Verification items for the finished model (mm, model axes). A direction names the side the tool comes from. Give positions to 0.01 mm unless a question says otherwise; leave off trailing zeros. Order: outer loops, then holes, each group sorted by start corner. A loop starts at its lowest first (then second) coordinate and runs counter-clockwise, first axis right, second up. Notation, with made-up numbers: (89, 36.5) -> (107, 36.5) arc R22 ccw to (107, 43.5) -> close; hole circle Ø2 at (84, 49.5). An arc over 180 degrees is marked (long way). Return JSON: item names as keys, results as strings. Group by question number.
(1) Depth check by flat-ended pin: pin 1 Ø6 at (x, y) = (32, -4) entering from -Z; pin 2 Ø4 at (x, y) = (51, -23) entering from +Z; pin 3 Ø10 at (x, z) = (38.5, 26) entering from -Y; pin 4 Ø4 at (y, z) = (-9, 34) entering from -X. Enter the tip coordinate at first touch or a pass-through.
(2) Cross-section at C-C on y = -25. Enter the section's corners in (x, z), then the cut area to 3 significant figures.
(3) Tool access check on faces 1 (the face through (12, -17, 2.54)), 2 (the face through (58, 0, 49)). Record the directions out of +Z, -Z, +X, -X, +Y, -Y that give a thin tool (end or side, any length) a straight path to the whole face; none if there is none.
(4) Cross-section at B-B on z = 54. Enter the section's corners in (x, y), then the cut area to 3 significant figures.
(5) Release check for a two-part mould opening along X. For faces 3 (the face through (58, -35, 49)), 4 (the face through (2.3, -17.3, 1.9)), 5 (the face through (66.861, -17.255, 52.706)) record: pulls with the +X half, pulls with the -X half, needs draft (parallel to the pull), parting line crosses it, or undercut.
(6) Cross-section at D-D on z = 22. Enter the section's corners in (x, y).
(7) Thickness scan on line 1 along Y through (x, z) = (15, 1.8); line 2 along Z through (x, y) = (13, -2.5); line 3 along X through (y, z) = (-27, 51). Record the ranges inside material, lowest first.
(8) Cross-section at A-A on x = 15. Enter the section's corners in (y, z).
from build123d import *

# Parameters (mm, degrees)
F1_DEPTH    = 35
F2_T1_DEPTH = 35
F2_T3_DEPTH = 60.4
F2_T5_DEPTH = 62.0452734599
F3_R        = 2.5
F4_DEPTH    = 61.0006540296


# Not quite as in the source:
# - a fillet or chamfer that OpenCascade refuses, or shapes differently, is made with other operations: its cross-section is extruded or revolved along the edge and cut away or added


with BuildPart() as f1:
    # F0 (on Front) → F1 (new body)
    with BuildSketch(Plane.XZ):
        with BuildLine():
            Line((0, 2.54), (0, 0))
            Line((0, 0), (25, 0))
            ThreePointArc((25, 0), (67.7784437716, 53.0927080046), (135.550785483, 45.6267456604))
            Line((135.550785483, 45.6267456604), (137.0076696313, 47.7073918529))
            ThreePointArc((137.0076696313, 47.7073918529), (67.7975373338, 55.8400571127), (22.9055940849, 2.54))
            Line((22.9055940849, 2.54), (0, 2.54))
        make_face()
    extrude(amount=F1_DEPTH)

    # F2: fillet of radius 6.35 on 3 edges, made by hand

    # F2_s2 → F2_t1 (join)
    with BuildSketch(Plane.XZ):
        with BuildLine():
            ThreePointArc((17.9186335189, 2.54), (21.7605713102, 3.8341109577), (24.0365583001, 7.1889719661))
            ThreePointArc((24.0365583001, 7.1889719661), (23.4332372688, 4.8736911297), (22.9055940849, 2.54))
            Line((22.9055940849, 2.54), (17.9186335189, 2.54))
        make_face()
    extrude(amount=F2_T1_DEPTH)

    # F2_s4 → F2_t3 (cut)
    with BuildSketch(Plane.XZ.offset(-12.7)):
        with BuildLine():
            ThreePointArc((5.08, 2.54), (2.2401936686, 1.8696126628), (0, 0))
            Line((0, 0), (0, 2.54))
            Line((0, 2.54), (5.08, 2.54))
        make_face()
    extrude(amount=F2_T3_DEPTH, mode=Mode.SUBTRACT)

    # F2_s6 → F2_t5 (cut)
    with BuildSketch(Plane.XZ.offset(-13.52263673)):
        with BuildLine():
            ThreePointArc((132.4656708106, 50.6447579134), (134.6252880595, 48.5151252309), (135.550785483, 45.6267456604))
            Line((135.550785483, 45.6267456604), (137.0076696313, 47.7073918529))
            ThreePointArc((137.0076696313, 47.7073918529), (134.7637005445, 49.2178714094), (132.4656708106, 50.6447579134))
        make_face()
    extrude(amount=F2_T5_DEPTH, mode=Mode.SUBTRACT)

    # F3 (on face) → F4 (cut, through all)
    with BuildSketch(Plane(origin=(0, 0, 0), x_dir=(1, 0, 0), z_dir=(0, 0, -1))):
        with Locations((15, 17.5375)):
            Circle(F3_R)
    extrude(amount=-F4_DEPTH, mode=Mode.SUBTRACT)


solid = f1.part
Verdict:
{
 "1": {"pin 1": "z = 13.94", "pin 2": "z = 47.92", "pin 3": "y = -35", "pin 4": "x = 36.35"},
 "2": {"outline": "(0, 0) -> (25, 0) arc R70.96 cw to (135.55, 45.63) arc R6.35 ccw to (132.47, 50.64) arc R73.5 ccw to (24.04, 7.19) arc R6.35 cw to (17.92, 2.54) -> (5.08, 2.54) arc R6.35 ccw to start", "area": "423 mm²"},
 "3": {"face 1": "+Z, -X, +Y, -Y", "face 2": "+Z, -Z, +X, -X, +Y"},
 "4": {"outline": "(63.55, -35) -> (70.09, -35) -> (70.09, 0) -> (63.55, 0) -> close; (119.61, -35) -> (126.15, -35) -> (126.15, 0) -> (119.61, 0) -> close", "area": "458 mm²"},
 "5": {"face 3": "needs draft", "face 4": "pulls with the -X half", "face 5": "undercut"},
 "6": {"outline": "(29.95, -35) -> (32.84, -35) -> (32.84, 0) -> (29.95, 0) -> close"},
 "7": {"line 1": "-35 to -20.04, -15.04 to 0", "line 2": "0 to 2.54", "line 3": "57.84 to 63.18, 126.52 to 131.86"},
 "8": {"outline": "(-35, 0) -> (-20.04, 0) -> (-20.04, 2.54) -> (-35, 2.54) -> close; (-15.04, 0) -> (0, 0) -> (0, 2.54) -> (-15.04, 2.54) -> close"}
}
